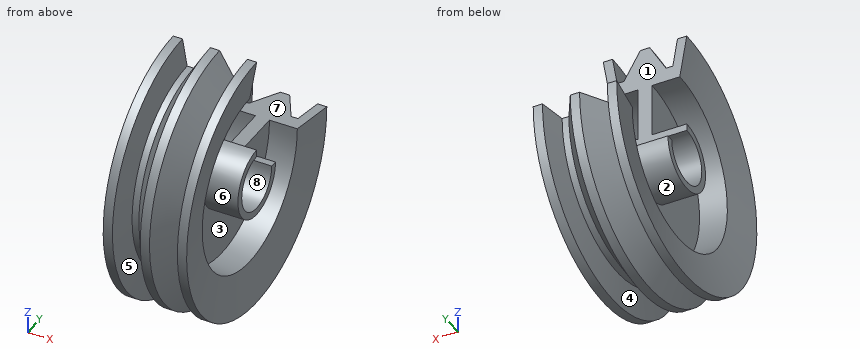
from build123d import *

# Parameters (mm, degrees)
REVOLVE5_ANGLE = 270


with BuildPart() as part:
    # Sketch1 → Revolve5 (revolve)
    with BuildSketch(Plane.XY):
        Polygon((-35.442504871, -11.710433312), (-35.442504871, -19.210433312), (54.557495129, -19.210433312), (54.557495129, -11.710433312), (17.057495129, -11.710433312), (17.057495129, 45.789566688), (47.057495129, 45.789566688), (54.557495129, 90.789566688), (44.557495129, 90.789566688), (39.557495129, 60.789566688), (32.265242588, 60.789566688), (14.567304664, 90.789573408), (4.557495129, 90.80620168), (-13.15025233, 60.789566688), (-20.442504871, 60.789566688), (-25.442504871, 90.789566688), (-35.442504871, 90.789566688), (-27.942504871, 45.789566688), (2.057495129, 45.789566688), (2.057495129, -11.710433312), align=None)
    revolve(axis=Axis((-35.442504871, -49.210433312, 0), (-1, 0, 0)), revolution_arc=REVOLVE5_ANGLE)


solid = part.part
The listing builds one solid part. Answer for the finished solid, in the listing's coordinates (mm). Face numbers are marked on the shaded views. A direction names the side the tool comes from. Round coordinates to 2 decimals unless told otherwise and drop trailing zeros. Order: outer loops, then holes, each group sorted by start corner. A loop starts at its lowest first (then second) coordinate and runs counter-clockwise, first axis right, second up. Notation, with made-up numbers: (-16.5, -28.75) - (-7.5, -28.75) arc R16 ccw to (-7.5, -6.75) - close; hole circle Ø7 at (26, -18.5). An arc over 180 degrees is marked (long way). Write item = value, one per line. Start each with the question number.
1) For a pull along Z with two mould halves and no side action, classify the marked faces 5, 6, 7 and 8 as released by +Z, released by -Z, zero draft, split by the parting line, or undercut.
2) Section A-A, the plane y = 64.5 is taken. Count the separate pieces of the cut face and the enclosed holes in it, plus the area to 3 significant figures.
3) Section B-B, the plane x = 8 is taken. Write down the section's boundary in (y, z).
4) Straight lines are drawn through the part: L1, parallel to Y at x = 36, z = -1; L2, parallel to X at y = 79, z = -23; L3, parallel to X at y = -106, z = 33.5. For each, find the intervals that lie inside material, in ascending order.
5) For the marked faces 1, 2, 3 and 4, determine the directions among +Z, -Z, +X, -X, +Y, -Y from which every point of the face is accessible in a straight line to the end or side of a thin tool.
6) Given pin 1 (1.5 mm diameter, centred on y = 51, z = -62.5, fed in from -X); pin 2 (12 mm diameter, centred on x = 19, y = 1.5, fed in from +Z); pin 3 (1 mm diameter, centred on x = -15, y = 17.5, fed in from +Z), each flat-ended and moving along its own axis, determine where each tip first touches the part or whether it passes through.
Results list:
q1.face_5 = split by the parting line
q1.face_6 = undercut
q1.face_7 = released by +Z
q1.face_8 = undercut
q2.separate_pieces = 3
q2.enclosed_holes = 0
q2.area = 4,110 mm^2
q3.outline = (-49.21, 30) - (-49.21, 140.01) arc R140.01 ccw (long way) to (90.8, 0) - (-19.21, 0) arc R30 cw (long way) to start
q4.L1 = -159.21 to -144.21, -86.7 to -79.19, -19.23 to -11.72, 45.78 to 60.79
q4.L2 = -33.82 to -23.82, -1.2 to 20.31, 42.93 to 52.93
q4.L3 = 2.06 to 17.06
q5.face_1 = +Z, +X, -X, +Y
q5.face_2 = -X
q5.face_3 = +X
q5.face_4 = none
q6.pin_1 = -31.92
q6.pin_2 = 0
q6.pin_3 = -67.14
